Could you check a few things on this model? Use its own coordinates, in mm. A direction names the side the tool comes from. Coordinates: 2 decimals unless noted, no trailing zeros. Write each loop counter-clockwise with the first axis right and the second up, starting at its lowest first coordinate (ties: lowest second). Pieces come first, ordered by that corner, then holes. Notation, with made-up numbers: (-18, 72.5) - (11, 72.5) arc R21 ccw to (11, 85.5) - close; hole circle Ø5 at (48, 11.5). An arc over 180 degrees is marked (long way). Write item = value, one per line. Start each with the question number.
```python
from build123d import *

# Parameters (mm, degrees)
F1_DEPTH = 7.45


with BuildPart() as f1:
    # F0 (on Front) → F1 (new body, symmetric)
    with BuildSketch(Plane.XZ):
        with BuildLine():
            Line((-8.5, -30.0970471648), (-4.3, -36.825))
            Line((-4.3, -36.825), (-4.3, -40.625))
            ThreePointArc((-4.3, -40.625), (-4.0071067812, -41.3321067812), (-3.3, -41.625))
            Line((-3.3, -41.625), (7.45, -41.625))
            Line((7.45, -41.625), (7.45, -44.825))
            Line((7.45, -44.825), (6.7, -44.825))
            Line((6.7, -44.825), (6.7, -47.025))
            Line((6.7, -47.025), (10.2, -47.025))
            Line((10.2, -47.025), (10.2, -38.425))
            ThreePointArc((10.2, -38.425), (9.9071067812, -37.7178932188), (9.2, -37.425))
            Line((9.2, -37.425), (0, -37.425))
            Line((0, -37.425), (0, 37.425))
            Line((0, 37.425), (8.4, 37.425))
            Line((8.4, 37.425), (8.4, 33.425))
            ThreePointArc((8.4, 33.425), (8.6928932188, 32.7178932188), (9.4, 32.425))
            Line((9.4, 32.425), (9.7, 32.425))
            ThreePointArc((9.7, 32.425), (10.4071067812, 32.7178932188), (10.7, 33.425))
            Line((10.7, 33.425), (10.7, 40.875))
            Line((10.7, 40.875), (12.0584372697, 42.3947607825))
            ThreePointArc((12.0584372697, 42.3947607825), (12.5542284753, 43.4993517405), (12.3218441058, 44.6875973417))
            Line((12.3218441058, 44.6875973417), (9.6272657122, 49.6124442137))
            ThreePointArc((9.6272657122, 49.6124442137), (8.7116734449, 51.9351925206), (8.4, 54.4123539124))
            Line((8.4, 54.4123539124), (8.4, 57.375))
            ThreePointArc((8.4, 57.375), (8.1071067812, 58.0821067812), (7.4, 58.375))
            Line((7.4, 58.375), (7.1, 58.375))
            ThreePointArc((7.1, 58.375), (6.3928932188, 58.0821067812), (6.1, 57.375))
            Line((6.1, 57.375), (6.1, 54.4123539124))
            ThreePointArc((6.1, 54.4123539124), (6.4116734449, 51.9351925206), (7.3272657122, 49.6124442137))
            Line((7.3272657122, 49.6124442137), (10.0218441058, 44.6875973417))
            ThreePointArc((10.0218441058, 44.6875973417), (10.2542284753, 43.4993517405), (9.7584372697, 42.3947607825))
            Line((9.7584372697, 42.3947607825), (8.4, 40.875))
            Line((8.4, 40.875), (-3.3, 40.875))
            ThreePointArc((-3.3, 40.875), (-4.0071067812, 40.5821067812), (-4.3, 39.875))
            Line((-4.3, 39.875), (-4.3, 33.875))
            Line((-4.3, 33.875), (-8.5, 29.375))
            Line((-8.5, 29.375), (-8.5, 20.075))
            Line((-8.5, 20.075), (-13.95, 20.075))
            Line((-13.95, 20.075), (-13.95, 29.375))
            Line((-13.95, 29.375), (-16.45, 29.375))
            ThreePointArc((-16.45, 29.375), (-17.8642135624, 28.7892135624), (-18.45, 27.375))
            Line((-18.45, 27.375), (-18.45, 13.875))
            Line((-18.45, 13.875), (-8.5, 6.6029528352))
            Line((-8.5, 6.6029528352), (-8.5, -30.0970471648))
        make_face()
    extrude(amount=F1_DEPTH, both=True)


solid = f1.part
```
1) Suppose I cut it at C-C on z = 1.5. Please give me the cut outline in (x, y).
2) Thinking about a two-plate mould opening in X: for faces 5 (the flat face through (4, 0, 37.425)), 6 (the cylindrical face through (12.55, -0.1, 43.48)), 7 (the flat face through (-15, 0, 29.375)), which applies, +X half, -X half, draft (parallel to the pull), parting line (faces both ways), or undercut?
3) Suppose I cut it at B-B on z = 26. Please give me the cut outline in (x, y).
4) Which directions (+Z, -Z, +X, -X, +Y, -Y) give clear straight access to the entire face, cutting with the end or side of a thin tool? Please do faces 1 (the flat face through (-4.3, 0, -39)), 2 (the flat face through (3, 0, 40.875)), 3 (the flat face through (6.1, 0, 56)), 4 (the flat face through (10.2, 0, -43)).
5) For P1, Ø6, axis at y = -2.5, z = -28, coming from the +X side; P2, Ø2.5, axis at y = 0.5, z = -46, coming from the -X side; P3, Ø10, axis at x = 6.5, z = 11.5, coming from the +Y side; P4, Ø2, axis at x = -2.5, y = -2.5, coming from the +Z side (3 decimals), each with a flat end and sliding along its axis, tell me the tip position at first contact or that it passes through.
6) Suppose I cut it at A-A on x = 1. Please give me the cut outline in (y, z) (3 decimals), plus the area to 3 significant figures.
7) If I drill on probe 1 along Z at (x, y) = (3.5, -2) (3 decimals); probe 2 along Z at (x, y) = (8, 6.5) (3 decimals); probe 3 along X at (y, z) = (-3, 21.5), over which ranges is the centre line in solid material (lowest first)? Write a range as [from, to].
Reply:
q1.outline = (-8.5, -7.45) - (0, -7.45) - (0, 7.45) - (-8.5, 7.45) - close
q2.face_5 = undercut
q2.face_6 = +X half
q2.face_7 = draft
q3.outline = (-18.45, -7.45) - (-13.95, -7.45) - (-13.95, 7.45) - (-18.45, 7.45) - close; (-8.5, -7.45) - (0, -7.45) - (0, 7.45) - (-8.5, 7.45) - close
q4.face_1 = -Z, -X, +Y, -Y
q4.face_2 = -X, +Y, -Y
q4.face_3 = +Z, -X, +Y, -Y
q4.face_4 = -Z, +X, +Y, -Y
q5.P1 = 0
q5.P2 = 6.7
q5.P3 = through
q5.P4 = 40.875
q6.outline = (-7.45, -41.625) - (7.45, -41.625) - (7.45, -37.425) - (-7.45, -37.425) - close; (-7.45, 37.425) - (7.45, 37.425) - (7.45, 40.875) - (-7.45, 40.875) - close
q6.area = 114 mm^2
q7.probe_1 = [-41.625, -37.425], [37.425, 40.875]
q7.probe_2 = [-47.025, -37.425], [37.425, 40.875], [48.383, 58.175]
q7.probe_3 = [-18.45, -13.95], [-8.5, 0]
